The model under review builds one solid part; all positions refer to its coordinate system, in mm. A direction names the side the tool comes from. Coordinates: 2 decimals unless noted, no trailing zeros. Loops run counter-clockwise (first coordinate to the right, second up) from the corner with the lowest first, then second, coordinate; pieces in that order, holes last. Notation, with made-up numbers: (-23, 60.5) - (5, 60.5) arc R10 cw to (5, 71.5) - close; hole circle Ø4 at (73.25, 87). An arc over 180 degrees is marked (long way). Answer in a Markdown table with one row per item. Add a question column.
(1) We need section A-A on x = -228.5. Write out the cut boundary in (y, z), plus the area to 3 significant figures.
(2) For line 1 along Z through (x, y) = (-125, 12.25); line 2 along X through (y, z) = (14.5, 40); line 3 along X through (y, z) = (10, 62), list the stretches that pass through material, from the lowest coordinate up.
(3) We need section B-B on y = 11.25. Give the number of separate pieces and of enclosed holes in the cut face, plus the area to 3 significant figures.
(4) Machinability: for faces 1 (the flat face through (-300, 10, 70)), 2 (the flat face through (290, 10, 40)), which of the approach directions +Z, -Z, +X, -X, +Y, -Y give a long, thin tool a straight path to every point of the face, cutting with its end or side? Answer none if there is none.
(5) Mouldability with a two-part tool opening along X and no side actions: class faces 3 (the flat face through (-310, 10, 29)), 4 (the flat face through (-1, 0, 6)), 5 (the flat face through (-4, 10, 10)) as +X half, -X half, draft (parallel to the pull), parting line (faces both ways), or undercut.
(6) For P1, Ø3, axis at x = -299.79, z = 60, coming from the +Y side; P2, Ø8, axis at x = 79, y = 17.5, coming from the +Z side, all flat-tipped, find the tip position at first contact; note any pin that passes through.
from build123d import *

# Parameters (mm, degrees)
SKETCH_1_W          = 580
SKETCH_1_H          = 20
EXTRUDE_1_DEPTH     = 20
CUT_EXTRUDE_1_REACH = 320.434
SKETCH_2_R          = 1.75
CUT_EXTRUDE_2_REACH = 320.434
SKETCH_4_R          = 1.75
CUT_EXTRUDE_3_REACH = 320.434
SKETCH_3_R          = 1.75


with BuildPart() as part:
    # 草图1 → 凸台-拉伸1 (new body)
    with BuildSketch(Plane(origin=(0, 0, 0), x_dir=(1, 0, 0), z_dir=(0, 1, 0))):
        Rectangle(SKETCH_1_W, SKETCH_1_H)
        Polygon((-290, -70), (-290, -10), (-290, 10), (-310, 10), (-310, -70), align=None)
        Polygon((290, 10), (290, -10), (290, -70), (310, -70), (310, 10), align=None)
    extrude(amount=EXTRUDE_1_DEPTH)

    # 草图2 → 切除-拉伸1 (cut, up to next)
    with BuildSketch(Plane(origin=(0, 20, 0), x_dir=(1, 0, 0), z_dir=(0, 1, 0)), mode=Mode.PRIVATE) as cut_extrude_1_sk1:
        with Locations(Location((-299.785666285, -40, 0), (0, 0, 270))):
            Circle(SKETCH_2_R)
    cut_extrude_1_tool1 = extrude(cut_extrude_1_sk1.sketch, amount=-CUT_EXTRUDE_1_REACH, mode=Mode.PRIVATE) & part.part
    # 草图2 → 切除-拉伸1 (cut, up to next)
    with BuildSketch(Plane(origin=(0, 20, 0), x_dir=(1, 0, 0), z_dir=(0, 1, 0)), mode=Mode.PRIVATE) as cut_extrude_1_sk2:
        with Locations(Location((-299.785666285, -60, 0), (0, 0, 270))):
            Circle(SKETCH_2_R)
    cut_extrude_1_tool2 = extrude(cut_extrude_1_sk2.sketch, amount=-CUT_EXTRUDE_1_REACH, mode=Mode.PRIVATE) & part.part
    # 草图2 → 切除-拉伸1 (cut, up to next)
    with BuildSketch(Plane(origin=(0, 20, 0), x_dir=(1, 0, 0), z_dir=(0, 1, 0)), mode=Mode.PRIVATE) as cut_extrude_1_sk3:
        with Locations(Location((-299.785666285, -20, 0), (0, 0, 270))):
            Circle(SKETCH_2_R)
    cut_extrude_1_tool3 = extrude(cut_extrude_1_sk3.sketch, amount=-CUT_EXTRUDE_1_REACH, mode=Mode.PRIVATE) & part.part
    # 草图2 → 切除-拉伸1 (cut, up to next)
    with BuildSketch(Plane(origin=(0, 20, 0), x_dir=(1, 0, 0), z_dir=(0, 1, 0)), mode=Mode.PRIVATE) as cut_extrude_1_sk4:
        with Locations(Location((-299.785666285, 0, 0), (0, 0, 270))):
            Circle(SKETCH_2_R)
    cut_extrude_1_tool4 = extrude(cut_extrude_1_sk4.sketch, amount=-CUT_EXTRUDE_1_REACH, mode=Mode.PRIVATE) & part.part
    add(cut_extrude_1_tool1.solids().sort_by_distance((-299.785666, 20, 40))[0], mode=Mode.SUBTRACT)
    add(cut_extrude_1_tool2.solids().sort_by_distance((-299.785666, 20, 60))[0], mode=Mode.SUBTRACT)
    add(cut_extrude_1_tool3.solids().sort_by_distance((-299.785666, 20, 20))[0], mode=Mode.SUBTRACT)
    add(cut_extrude_1_tool4.solids().sort_by_distance((-299.785666, 20, 0))[0], mode=Mode.SUBTRACT)

    # 草图4 → 切除-拉伸2 (cut, up to next)
    with BuildSketch(Plane(origin=(0, 20, 0), x_dir=(1, 0, 0), z_dir=(0, 1, 0)), mode=Mode.PRIVATE) as cut_extrude_2_sk1:
        with Locations(Location((-125, 0, 0), (0, 0, 270))):
            Circle(SKETCH_4_R)
    cut_extrude_2_tool1 = extrude(cut_extrude_2_sk1.sketch, amount=-CUT_EXTRUDE_2_REACH, mode=Mode.PRIVATE) & part.part
    # 草图4 → 切除-拉伸2 (cut, up to next)
    with BuildSketch(Plane(origin=(0, 20, 0), x_dir=(1, 0, 0), z_dir=(0, 1, 0)), mode=Mode.PRIVATE) as cut_extrude_2_sk2:
        with Locations(Location((-105, 0, 0), (0, 0, 270))):
            Circle(SKETCH_4_R)
    cut_extrude_2_tool2 = extrude(cut_extrude_2_sk2.sketch, amount=-CUT_EXTRUDE_2_REACH, mode=Mode.PRIVATE) & part.part
    # 草图4 → 切除-拉伸2 (cut, up to next)
    with BuildSketch(Plane(origin=(0, 20, 0), x_dir=(1, 0, 0), z_dir=(0, 1, 0)), mode=Mode.PRIVATE) as cut_extrude_2_sk3:
        with Locations(Location((-145, 0, 0), (0, 0, 270))):
            Circle(SKETCH_4_R)
    cut_extrude_2_tool3 = extrude(cut_extrude_2_sk3.sketch, amount=-CUT_EXTRUDE_2_REACH, mode=Mode.PRIVATE) & part.part
    # 草图4 → 切除-拉伸2 (cut, up to next)
    with BuildSketch(Plane(origin=(0, 20, 0), x_dir=(1, 0, 0), z_dir=(0, 1, 0)), mode=Mode.PRIVATE) as cut_extrude_2_sk4:
        with Locations(Location((105, 0, 0), (0, 0, 270))):
            Circle(SKETCH_4_R)
    cut_extrude_2_tool4 = extrude(cut_extrude_2_sk4.sketch, amount=-CUT_EXTRUDE_2_REACH, mode=Mode.PRIVATE) & part.part
    # 草图4 → 切除-拉伸2 (cut, up to next)
    with BuildSketch(Plane(origin=(0, 20, 0), x_dir=(1, 0, 0), z_dir=(0, 1, 0)), mode=Mode.PRIVATE) as cut_extrude_2_sk5:
        with Locations(Location((125, 0, 0), (0, 0, 270))):
            Circle(SKETCH_4_R)
    cut_extrude_2_tool5 = extrude(cut_extrude_2_sk5.sketch, amount=-CUT_EXTRUDE_2_REACH, mode=Mode.PRIVATE) & part.part
    # 草图4 → 切除-拉伸2 (cut, up to next)
    with BuildSketch(Plane(origin=(0, 20, 0), x_dir=(1, 0, 0), z_dir=(0, 1, 0)), mode=Mode.PRIVATE) as cut_extrude_2_sk6:
        with Locations(Location((145, 0, 0), (0, 0, 270))):
            Circle(SKETCH_4_R)
    cut_extrude_2_tool6 = extrude(cut_extrude_2_sk6.sketch, amount=-CUT_EXTRUDE_2_REACH, mode=Mode.PRIVATE) & part.part
    add(cut_extrude_2_tool1.solids().sort_by_distance((-125, 20, 0))[0], mode=Mode.SUBTRACT)
    add(cut_extrude_2_tool2.solids().sort_by_distance((-105, 20, 0))[0], mode=Mode.SUBTRACT)
    add(cut_extrude_2_tool3.solids().sort_by_distance((-145, 20, 0))[0], mode=Mode.SUBTRACT)
    add(cut_extrude_2_tool4.solids().sort_by_distance((105, 20, 0))[0], mode=Mode.SUBTRACT)
    add(cut_extrude_2_tool5.solids().sort_by_distance((125, 20, 0))[0], mode=Mode.SUBTRACT)
    add(cut_extrude_2_tool6.solids().sort_by_distance((145, 20, 0))[0], mode=Mode.SUBTRACT)

    # 草图3 → 切除-拉伸3 (cut, up to next)
    with BuildSketch(Plane.XZ, mode=Mode.PRIVATE) as cut_extrude_3_sk1:
        with Locations(Location((180, 0, 0), (0, 0, 270))):
            Circle(SKETCH_3_R)
    cut_extrude_3_tool1 = extrude(cut_extrude_3_sk1.sketch, amount=-CUT_EXTRUDE_3_REACH, mode=Mode.PRIVATE) & part.part
    # 草图3 → 切除-拉伸3 (cut, up to next)
    with BuildSketch(Plane.XZ, mode=Mode.PRIVATE) as cut_extrude_3_sk2:
        with Locations(Location((280, 0, 0), (0, 0, 270))):
            Circle(SKETCH_3_R)
    cut_extrude_3_tool2 = extrude(cut_extrude_3_sk2.sketch, amount=-CUT_EXTRUDE_3_REACH, mode=Mode.PRIVATE) & part.part
    # 草图3 → 切除-拉伸3 (cut, up to next)
    with BuildSketch(Plane.XZ, mode=Mode.PRIVATE) as cut_extrude_3_sk3:
        with Locations(Location((260, 0, 0), (0, 0, 270))):
            Circle(SKETCH_3_R)
    cut_extrude_3_tool3 = extrude(cut_extrude_3_sk3.sketch, amount=-CUT_EXTRUDE_3_REACH, mode=Mode.PRIVATE) & part.part
    # 草图3 → 切除-拉伸3 (cut, up to next)
    with BuildSketch(Plane.XZ, mode=Mode.PRIVATE) as cut_extrude_3_sk4:
        with Locations(Location((-280, 0, 0), (0, 0, 270))):
            Circle(SKETCH_3_R)
    cut_extrude_3_tool4 = extrude(cut_extrude_3_sk4.sketch, amount=-CUT_EXTRUDE_3_REACH, mode=Mode.PRIVATE) & part.part
    # 草图3 → 切除-拉伸3 (cut, up to next)
    with BuildSketch(Plane.XZ, mode=Mode.PRIVATE) as cut_extrude_3_sk5:
        with Locations(Location((-260, 0, 0), (0, 0, 270))):
            Circle(SKETCH_3_R)
    cut_extrude_3_tool5 = extrude(cut_extrude_3_sk5.sketch, amount=-CUT_EXTRUDE_3_REACH, mode=Mode.PRIVATE) & part.part
    # 草图3 → 切除-拉伸3 (cut, up to next)
    with BuildSketch(Plane.XZ, mode=Mode.PRIVATE) as cut_extrude_3_sk6:
        with Locations(Location((-180, 0, 0), (0, 0, 270))):
            Circle(SKETCH_3_R)
    cut_extrude_3_tool6 = extrude(cut_extrude_3_sk6.sketch, amount=-CUT_EXTRUDE_3_REACH, mode=Mode.PRIVATE) & part.part
    add(cut_extrude_3_tool1.solids().sort_by_distance((180, 0, 0))[0], mode=Mode.SUBTRACT)
    add(cut_extrude_3_tool2.solids().sort_by_distance((280, 0, 0))[0], mode=Mode.SUBTRACT)
    add(cut_extrude_3_tool3.solids().sort_by_distance((260, 0, 0))[0], mode=Mode.SUBTRACT)
    add(cut_extrude_3_tool4.solids().sort_by_distance((-280, 0, 0))[0], mode=Mode.SUBTRACT)
    add(cut_extrude_3_tool5.solids().sort_by_distance((-260, 0, 0))[0], mode=Mode.SUBTRACT)
    add(cut_extrude_3_tool6.solids().sort_by_distance((-180, 0, 0))[0], mode=Mode.SUBTRACT)


solid = part.part
Outcome:
| question | item | result |
|---|---|---|
| 1 | outline | (0, -10) - (20, -10) - (20, 10) - (0, 10) - close |
| 1 | area | 400 mm² |
| 2 | line 1 | -10 to -1.75, 1.75 to 10 |
| 2 | line 2 | -310 to -301.54, -298.04 to -290, 290 to 310 |
| 2 | line 3 | -310 to -290, 290 to 310 |
| 3 | separate pieces | 1 |
| 3 | enclosed holes | 16 |
| 3 | area | 14,600 mm² |
| 4 | face 1 | +Z, +X, -X, +Y, -Y |
| 4 | face 2 | +Z, +Y, -Y |
| 5 | face 3 | -X half |
| 5 | face 4 | draft |
| 5 | face 5 | undercut |
| 6 | P1 | through |
| 6 | P2 | z = 10 |
